from build123d import *

# Parameters (mm, degrees)
BOSS_EXTRUDE1_DEPTH      = 25
BOSS_EXTRUDE1_DEPTH_BACK = 25
SKETCH8_R                = 37
SKETCH8_W                = 55
SKETCH8_H                = 30
CUT_EXTRUDE1_DEPTH       = 20
CUT_EXTRUDE1_DEPTH_BACK  = 35
CUT_EXTRUDE2_DEPTH       = 65
CUT_EXTRUDE4_DEPTH       = 113.525762116
SKETCH16_R               = 40.190590084
SKETCH16_R_2             = 37
BOSS_EXTRUDE3_DEPTH      = 3


with BuildPart() as part:
    # Sketch8 → Boss-Extrude1 (new, two sides: drawn at the far end of the back side and taken through both)
    with BuildSketch(Plane(origin=(0, 0, 0), x_dir=(1, 0, 0), z_dir=(0, 1, 0)).offset(-BOSS_EXTRUDE1_DEPTH_BACK)):
        with BuildLine():
            Line((-13.333333333, 97.657806344), (-40, 97.657806344))
            ThreePointArc((-40, 97.657806344), (-47.071067812, 94.728874155), (-50, 87.657806344))
            Line((-50, 87.657806344), (-50, 8.828903172))
            Line((-50, 8.828903172), (-50, -70))
            ThreePointArc((-50, -70), (-47.071067812, -77.071067812), (-40, -80))
            Line((-40, -80), (40, -80))
            ThreePointArc((40, -80), (47.071067812, -77.071067812), (50, -70))
            Line((50, -70), (50, 8.828903172))
            Line((50, 8.828903172), (50, 87.657806344))
            ThreePointArc((50, 87.657806344), (47.071067812, 94.728874155), (40, 97.657806344))
            Line((40, 97.657806344), (13.333333333, 97.657806344))
            Line((13.333333333, 97.657806344), (-13.333333333, 97.657806344))
        make_face()
        with Locations(Location((-0.034150482, 35.300694554, 0), (0, 0, 270))):
            Circle(SKETCH8_R, mode=Mode.SUBTRACT)
        with Locations((0, -38.093187293)):
            Rectangle(SKETCH8_W, SKETCH8_H, mode=Mode.SUBTRACT)
    extrude(amount=BOSS_EXTRUDE1_DEPTH + BOSS_EXTRUDE1_DEPTH_BACK)

    # Sketch14 → Cut-Extrude1 (cut, two sides: drawn at the far end of the back side and taken through both)
    with BuildSketch(Plane(origin=(0, 0, 0), x_dir=(1, 0, 0), z_dir=(0, 1, 0)).offset(-CUT_EXTRUDE1_DEPTH_BACK)):
        with BuildLine():
            Line((-37.755307684, 94.843507168), (37.755307684, 94.843507168))
            ThreePointArc((37.755307684, 94.843507168), (44.826375496, 91.91457498), (47.755307684, 84.843507168))
            Line((47.755307684, 84.843507168), (47.755307684, -68.296492832))
            ThreePointArc((47.755307684, -68.296492832), (44.826375496, -75.367560643), (37.755307684, -78.296492832))
            Line((37.755307684, -78.296492832), (-37.755307684, -78.296492832))
            ThreePointArc((-37.755307684, -78.296492832), (-44.826375496, -75.367560643), (-47.755307684, -68.296492832))
            Line((-47.755307684, -68.296492832), (-47.755307684, 84.843507168))
            ThreePointArc((-47.755307684, 84.843507168), (-44.826375496, 91.91457498), (-37.755307684, 94.843507168))
        make_face()
    extrude(amount=CUT_EXTRUDE1_DEPTH + CUT_EXTRUDE1_DEPTH_BACK, mode=Mode.SUBTRACT)

    # Sketch15 → Cut-Extrude2 (cut)
    with BuildSketch(Plane(origin=(0, 0, 0), x_dir=(0, 0, -1), z_dir=(1, 0, 0))):
        with BuildLine():
            Line((63.260342579, -13.058175161), (7.260342579, -13.058175161))
            ThreePointArc((7.260342579, -13.058175161), (5.846129016, -13.643961598), (5.260342579, -15.058175161))
            Line((5.260342579, -15.058175161), (5.260342579, -17.199912978))
            ThreePointArc((5.260342579, -17.199912978), (5.846129016, -18.61412654), (7.260342579, -19.199912978))
            Line((7.260342579, -19.199912978), (63.260342579, -19.199912978))
            ThreePointArc((63.260342579, -19.199912978), (64.674556141, -18.61412654), (65.260342579, -17.199912978))
            Line((65.260342579, -17.199912978), (65.260342579, -15.058175161))
            ThreePointArc((65.260342579, -15.058175161), (64.674556141, -13.643961598), (63.260342579, -13.058175161))
        make_face()
    extrude(amount=CUT_EXTRUDE2_DEPTH, mode=Mode.SUBTRACT)

    # Sketch9 → Cut-Extrude4 (cut, through all)
    with BuildSketch(Plane.XY):
        with BuildLine():
            Line((3.499295318, -13.313051471), (-3.500704682, -13.313051471))
            ThreePointArc((-3.500704682, -13.313051471), (-3.854258072, -13.45949808), (-4.000704682, -13.813051471))
            Line((-4.000704682, -13.813051471), (-4.000704682, -14.813051471))
            ThreePointArc((-4.000704682, -14.813051471), (-3.854258072, -15.166604861), (-3.500704682, -15.313051471))
            Line((-3.500704682, -15.313051471), (3.499295318, -15.313051471))
            ThreePointArc((3.499295318, -15.313051471), (3.852848709, -15.166604861), (3.999295318, -14.813051471))
            Line((3.999295318, -14.813051471), (3.999295318, -13.813051471))
            ThreePointArc((3.999295318, -13.813051471), (3.852848709, -13.45949808), (3.499295318, -13.313051471))
        make_face()
    extrude(amount=CUT_EXTRUDE4_DEPTH, mode=Mode.SUBTRACT)

    # Sketch16 → Boss-Extrude3 (add)
    with BuildSketch(Plane(origin=(0, 25, 0), x_dir=(1, 0, 0), z_dir=(0, 1, 0))):
        with Locations(Location((-0.197566829, 35.094491393, 0), (0, 0, 270))):
            Circle(SKETCH16_R)
        with Locations(Location((-0.034150482, 35.300694554, 0), (0, 0, 270))):
            Circle(SKETCH16_R_2, mode=Mode.SUBTRACT)
    extrude(amount=BOSS_EXTRUDE3_DEPTH)


solid = part.part
Can you work these out from the model? Positions are in its coordinate system, mm. A direction names the side the tool comes from. Round coordinates to 2 decimals unless told otherwise and drop trailing zeros. Write each loop counter-clockwise with the first axis right and the second up, starting at its lowest first coordinate (ties: lowest second). Pieces come first, ordered by that corner, then holes. Notation, with made-up numbers: M 45,-5 L 99,-5 A21 cw 99,23 Z; hole C 83,69 d4. An arc over 180 degrees is marked long. Use a Markdown table: item, result.
Item 1: I want a section at C-C (z = 14.5). List the corners of the cut face in (x, y) for me.
Found:
| item | result |
|---|---|
| outline | M -50,-25 L -47.76,-25 L -47.76,20 L 47.76,20 L 47.76,-25 L 50,-25 L 50,25 L -50,25 Z |
Item 2: I want a section at B-B (y = -11). List the corners of the cut face in (x, z) for me, and give its area (3 significant figures).
Found:
| item | result |
|---|---|
| outline | M -50,-87.66 A10 ccw -40,-97.66 L 40,-97.66 A10 ccw 50,-87.66 L 50,70 A10 ccw 40,80 L -40,80 A10 ccw -50,70 Z; hole M -47.76,-84.84 A10 ccw -37.76,-94.84 L 37.76,-94.84 A10 ccw 47.76,-84.84 L 47.76,68.3 A10 ccw 37.76,78.3 L -37.76,78.3 A10 ccw -47.76,68.3 Z |
| area | 1,230 mm2 |
Item 3: Which directions (+Z, -Z, +X, -X, +Y, -Y) give clear straight access to the entire face, cutting with the end or side of a thin tool? Please do faces 1 (the face through (0, 22, 23.093)), 2 (the face through (-1, 25, 10)), 3 (the face through (1, -3, 78.296)).
Found:
| item | result |
|---|---|
| face 1 | +Y, -Y |
| face 2 | +Y |
| face 3 | -Y |
Item 4: I want a section at D-D (x = -31). List the corners of the cut face in (y, z) for me.
Found:
| item | result |
|---|---|
| outline | M -25,-97.66 L 25,-97.66 L 25,-60.91 L 28,-60.91 L 28,-55.55 L 20,-55.55 L 20,-94.84 L -25,-94.84 Z; M -25,78.3 L 20,78.3 L 20,-15.05 L 28,-15.05 L 28,-9.28 L 25,-9.28 L 25,80 L -25,80 Z |
Item 5: If I drill on line 1 along Z through (x, y) = (-17.5, -8.5); line 2 along X through (y, z) = (4.5, -76.5); line 3 along X through (y, z) = (24, 24.5), over which ranges is the centre line in solid material (lowest first)? Write a range as [from, to].
Found:
| item | result |
|---|---|
| line 1 | z = [-97.66, -94.84], [78.3, 80] |
| line 2 | x = [-50, -47.76], [47.76, 50] |
| line 3 | x = [-50, -27.5], [27.5, 50] |
Item 6: We'd pull the mould along X, two halves only. Please class faces 4 (the face through (-50, 0, -10)), 5 (the face through (0, 22, 53.093)), 6 (the face through (48, -25, -9)): released by +X, released by -X, zero draft, split by the parting line, or undercut.
Found:
| item | result |
|---|---|
| face 4 | released by -X |
| face 5 | undercut |
| face 6 | zero draft |
Item 7: For pin 1 Ø1.4 at (x, z) = (-0.5, 79) entering from +Y; pin 2 Ø1.5 at (x, z) = (-35.5, -18.5) entering from -Y; pin 3 Ø1.7 at (x, y) = (48.5, -16.5) entering from -Z, each with a flat end and sliding along its axis, tell me the tip position at first contact or that it passes through.
Found:
| item | result |
|---|---|
| pin 1 | stops at y = 25 |
| pin 2 | stops at y = 20 |
| pin 3 | stops at z = -94.1 |
Item 8: I want a section at A-A (x = 19). List the corners of the cut face in (y, z) for me, and give its area (3 significant figures).
Found:
| item | result |
|---|---|
| outline | M -25,-97.66 L 25,-97.66 L 25,-70.4 L 28,-70.4 L 28,-67.03 L 20,-67.03 L 20,-94.84 L -25,-94.84 Z; M -25,78.3 L 20,78.3 L 20,53.09 L 25,53.09 L 25,80 L -25,80 Z; M 20,-3.57 L 28,-3.57 L 28,0.21 L 25,0.21 L 25,23.09 L 20,23.09 Z |
| area | 646 mm2 |
